Can you work these out from the drawing? Everything is in mm from the part's minimum corner. A direction names the side the tool comes from. Coordinates: 2 decimals unless noted, no trailing zeros. Order: outer loops, then holes, each group sorted by start corner. A loop starts at its lowest first (then second) coordinate and runs counter-clockwise, first axis right, second up. Notation, with made-up numbers: (82.5, 55.25) - (107.5, 55.25) arc R24 cw to (107.5, 90.25) - close; hole circle Ø4 at (14.5, 47.5). An arc over 180 degrees is marked (long way). Use a Markdown table: item, result. Add a question column.
(1) I want a section at A-A (y = 11.1). List the corners of the cut face in (x, z) for me.
(2) For pin 1 Ø4 at (y, z) = (5, 2) entering from +X; pin 2 Ø6 at (x, z) = (6, 5.5) entering from +Y; pin 3 Ø6 at (y, z) = (18.5, 15) entering from +X, each with a flat end and sliding along its axis, tell me the tip position at first contact or that it passes through.
(3) On a 3-axis mill with a long thin cutter (end or side, diameter ignored), from which of +Z, -Z, +X, -X, +Y, -Y can I reach the whole of each face in a straight line? I mean the marked faces 4, 5 and 6. Say none if no direction works.
(4) I want a section at C-C (y = 3.75). List the corners of the cut face in (x, z) for me, and give its area (3 significant figures).
(5) I want a section at D-D (x = 3.1). List the corners of the cut face in (y, z) for me.
(6) If I drill on L1, parallel to Y at x = 11.1, z = 9; L2, parallel to X at y = 12, z = 6.5; L3, parallel to Y at x = 11.25, z = 2.25, over which ranges is the centre line in solid material (lowest first)? Write a range as [from, to].
(7) We'd pull the mould along Y, two halves only. Please class the marked faces 1, 2 and 3: pulls with the +Y half, pulls with the -Y half, needs draft (parallel to the pull), parting line crosses it, or undercut.
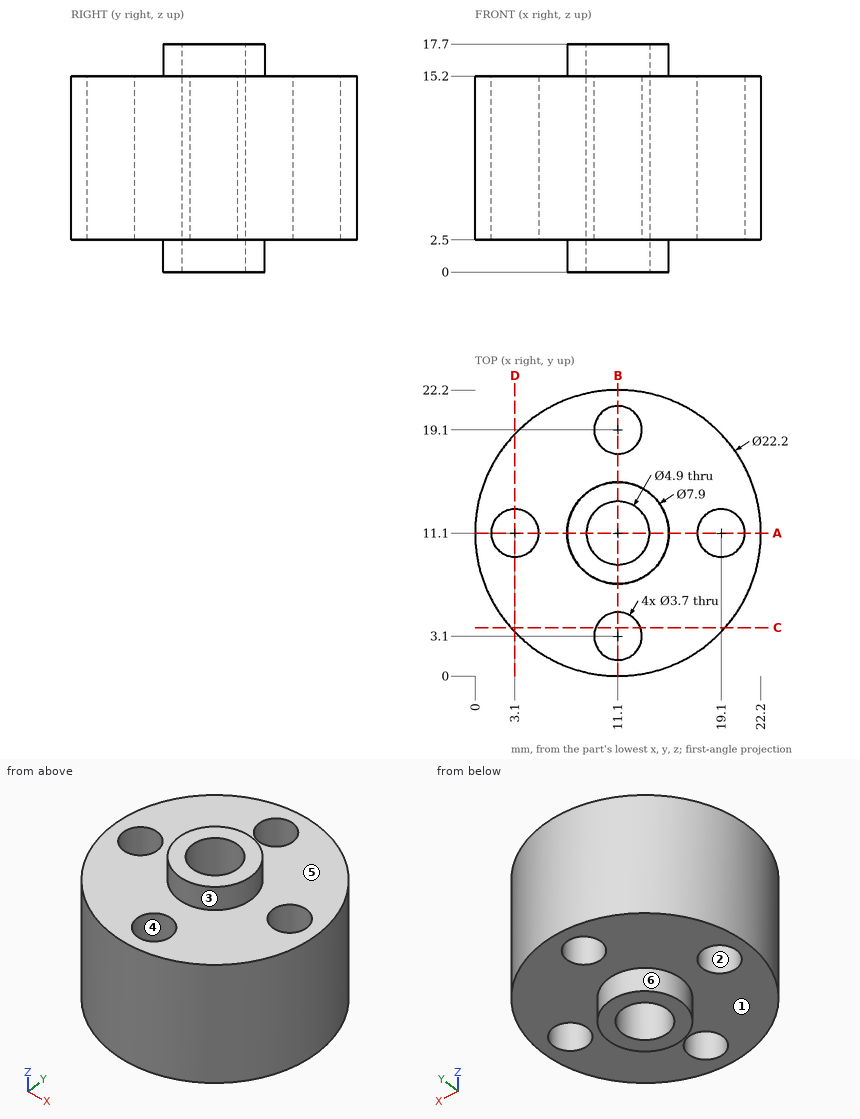
Answers follow:
| question | item | result |
|---|---|---|
| 1 | outline | (0, 2.5) - (1.25, 2.5) - (1.25, 15.2) - (0, 15.2) - close; (4.95, 2.5) - (7.15, 2.5) - (7.15, 0) - (8.65, 0) - (8.65, 17.7) - (7.15, 17.7) - (7.15, 15.2) - (4.95, 15.2) - close; (13.55, 0) - (15.05, 0) - (15.05, 2.5) - (17.25, 2.5) - (17.25, 15.2) - (15.05, 15.2) - (15.05, 17.7) - (13.55, 17.7) - close; (20.95, 2.5) - (22.2, 2.5) - (22.2, 15.2) - (20.95, 15.2) - close |
| 2 | pin 1 | stops at x = 21.39 |
| 2 | pin 2 | stops at y = 22 |
| 2 | pin 3 | stops at x = 21.29 |
| 3 | face 4 | +Z, -Z |
| 3 | face 5 | +Z |
| 3 | face 6 | -Z |
| 4 | outline | (2.78, 2.5) - (9.37, 2.5) - (9.37, 15.2) - (2.78, 15.2) - close; (12.83, 2.5) - (19.42, 2.5) - (19.42, 15.2) - (12.83, 15.2) - close |
| 4 | area | 167 mm² |
| 5 | outline | (3.41, 2.5) - (9.25, 2.5) - (9.25, 15.2) - (3.41, 15.2) - close; (12.95, 2.5) - (18.79, 2.5) - (18.79, 15.2) - (12.95, 15.2) - close |
| 6 | L1 | y = [0, 1.25], [4.95, 8.65], [13.55, 17.25], [20.95, 22.2] |
| 6 | L2 | x = [0.04, 1.48], [4.72, 8.82], [13.38, 17.48], [20.72, 22.16] |
| 6 | L3 | y = [7.15, 8.65], [13.55, 15.05] |
| 7 | face 1 | needs draft |
| 7 | face 2 | undercut |
| 7 | face 3 | parting line crosses it |
